Could you check a few things on this model? Use its own coordinates, in mm. A direction names the side the tool comes from. Give positions to 0.01 mm unless a question says otherwise; leave off trailing zeros. Write each loop counter-clockwise with the first axis right and the second up, starting at its lowest first coordinate (ties: lowest second). Pieces come first, ordered by that corner, then holes. Notation, with made-up numbers: (39.5, -32.5) -> (89.5, -32.5) arc R19 cw to (89.5, -5.5) -> close; hole circle Ø8 at (44.25, 2.5). An arc over 180 degrees is marked (long way). One line per question, with ' | ' between items.
from build123d import *
from build123d import SkipClean  # not in build123d's __all__

# Parameters (mm, degrees)
F0_R     = 2
F1_DEPTH = 2
F3_DEPTH = 1
F5_DEPTH = 5
F8_DEPTH = 8
F9_DEPTH = 8


with BuildPart() as f1:
    # F0 (on Top) → F1 (new body)
    with BuildSketch(Plane.XY):
        with BuildLine():
            ThreePointArc((-5, 0), (-3.5355339059, 3.5355339059), (0, 5))
            Line((0, 5), (0, 7))
            ThreePointArc((0, 7), (-4.9497474683, 4.9497474683), (-7, 0))
            Line((-7, 0), (-5, 0))
        make_face()
        with BuildLine():
            ThreePointArc((0, 5), (3.5355339059, 3.5355339059), (5, 0))
            Line((5, 0), (7, 0))
            ThreePointArc((7, 0), (4.9497474683, 4.9497474683), (0, 7))
            Line((0, 7), (0, 5))
        make_face()
        with BuildLine():
            Line((7, 0), (5, 0))
            ThreePointArc((5, 0), (3.5355339059, -3.5355339059), (0, -5))
            Line((0, -5), (0, -7))
            ThreePointArc((0, -7), (4.9497474683, -4.9497474683), (7, 0))
        make_face()
        with BuildLine():
            Line((0, -7), (0, -5))
            ThreePointArc((0, -5), (-3.5355339059, -3.5355339059), (-5, 0))
            Line((-5, 0), (-7, 0))
            ThreePointArc((-7, 0), (-4.9497474683, -4.9497474683), (0, -7))
        make_face()
        with BuildLine():
            ThreePointArc((0, -5), (3.5355339059, -3.5355339059), (5, 0))
            ThreePointArc((5, 0), (3.5355339059, 3.5355339059), (0, 5))
            ThreePointArc((0, 5), (-3.5355339059, 3.5355339059), (-5, 0))
            ThreePointArc((-5, 0), (-3.5355339059, -3.5355339059), (0, -5))
        make_face()
        Circle(F0_R, mode=Mode.SUBTRACT)
    extrude(amount=F1_DEPTH)

    # F2 (on face) → F3 (join)
    with BuildSketch(Plane.XY.offset(2)):
        with BuildLine():
            ThreePointArc((-5, 0), (-3.5355339059, 3.5355339059), (0, 5))
            Line((0, 5), (0, 7))
            ThreePointArc((0, 7), (-1.1928549598, 6.8976153158), (-2.3508156114, 6.5934562986))
            Line((-2.3508156114, 6.5934562986), (-6.5934562986, 2.3508156114))
            ThreePointArc((-6.5934562986, 2.3508156114), (-6.8976153158, 1.1928549598), (-7, 0))
            Line((-7, 0), (-5, 0))
        make_face()
        with BuildLine():
            Line((-6.5934562986, 2.3508156114), (-2.3508156114, 6.5934562986))
            ThreePointArc((-2.3508156114, 6.5934562986), (-4.9497474683, 4.9497474683), (-6.5934562986, 2.3508156114))
        make_face()
        with BuildLine():
            ThreePointArc((2.3508156114, -6.5934562986), (4.9497474683, -4.9497474683), (6.5934562986, -2.3508156114))
            Line((6.5934562986, -2.3508156114), (2.3508156114, -6.5934562986))
        make_face()
        with BuildLine():
            Line((7, 0), (5, 0))
            ThreePointArc((5, 0), (3.5355339059, -3.5355339059), (0, -5))
            Line((0, -5), (0, -7))
            ThreePointArc((0, -7), (1.1928549598, -6.8976153158), (2.3508156114, -6.5934562986))
            Line((2.3508156114, -6.5934562986), (6.5934562986, -2.3508156114))
            ThreePointArc((6.5934562986, -2.3508156114), (6.8976153158, -1.1928549598), (7, 0))
        make_face()
    with SkipClean():  # cleaning this boolean's faces spoils the solid; the shape is the same uncleaned
        extrude(amount=F3_DEPTH)

    # F4 (on face) → F5 (join)
    with BuildSketch(Plane.XY.offset(3)):
        with BuildLine():
            ThreePointArc((-5, 0), (-3.5355339059, 3.5355339059), (0, 5))
            Line((0, 5), (0, 7))
            ThreePointArc((0, 7), (-1.1928549598, 6.8976153158), (-2.3508156114, 6.5934562986))
            Line((-2.3508156114, 6.5934562986), (-6.5934562986, 2.3508156114))
            ThreePointArc((-6.5934562986, 2.3508156114), (-6.8976153158, 1.1928549598), (-7, 0))
            Line((-7, 0), (-5, 0))
        make_face()
        with BuildLine():
            Line((7, 0), (5, 0))
            ThreePointArc((5, 0), (3.5355339059, -3.5355339059), (0, -5))
            Line((0, -5), (0, -7))
            ThreePointArc((0, -7), (1.1928549598, -6.8976153158), (2.3508156114, -6.5934562986))
            Line((2.3508156114, -6.5934562986), (6.5934562986, -2.3508156114))
            ThreePointArc((6.5934562986, -2.3508156114), (6.8976153158, -1.1928549598), (7, 0))
        make_face()
    extrude(amount=F5_DEPTH)

    # F7 (on face) → F8 (join)
    with BuildSketch(Plane(origin=(4.472135955, -4.472135955, 0), x_dir=(0.7071067812, 0.7071067812, 0), z_dir=(0.7071067812, -0.7071067812, 0))):
        with BuildLine():
            Line((1.1523319194, 6.4602765995), (0, 5.5))
            Line((0, 5.5), (1.1523319194, 4.5397234005))
            ThreePointArc((1.1523319194, 4.5397234005), (1.4104073665, 4.9893621044), (1.5, 5.5))
            ThreePointArc((1.5, 5.5), (1.4104073665, 6.0106378956), (1.1523319194, 6.4602765995))
        make_face()
        with BuildLine():
            Line((0, 5.5), (-1.1523319194, 6.4602765995))
            ThreePointArc((-1.1523319194, 6.4602765995), (-1.5, 5.5), (-1.1523319194, 4.5397234005))
            Line((-1.1523319194, 4.5397234005), (0, 5.5))
        make_face()
        with BuildLine():
            ThreePointArc((1.1523319194, 6.4602765995), (0, 7), (-1.1523319194, 6.4602765995))
            Line((-1.1523319194, 6.4602765995), (0, 5.5))
            Line((0, 5.5), (1.1523319194, 6.4602765995))
        make_face()
        with BuildLine():
            Line((1.1523319194, 4.5397234005), (0, 5.5))
            Line((0, 5.5), (-1.1523319194, 4.5397234005))
            ThreePointArc((-1.1523319194, 4.5397234005), (0, 4), (1.1523319194, 4.5397234005))
        make_face()
    extrude(amount=F8_DEPTH)

    # F6 (on face) → F9 (join)
    with BuildSketch(Plane(origin=(-4.472135955, 4.472135955, 0), x_dir=(-0.7071067812, -0.7071067812, 0), z_dir=(-0.7071067812, 0.7071067812, 0))):
        with BuildLine():
            ThreePointArc((1.1523319194, 6.4602765995), (0, 7), (-1.1523319194, 6.4602765995))
            Line((-1.1523319194, 6.4602765995), (0, 5.5))
            Line((0, 5.5), (1.1523319194, 6.4602765995))
        make_face()
        with BuildLine():
            Line((1.1523319194, 6.4602765995), (0, 5.5))
            Line((0, 5.5), (1.1523319194, 4.5397234005))
            ThreePointArc((1.1523319194, 4.5397234005), (1.4104073665, 4.9893621044), (1.5, 5.5))
            ThreePointArc((1.5, 5.5), (1.4104073665, 6.0106378956), (1.1523319194, 6.4602765995))
        make_face()
        with BuildLine():
            Line((1.1523319194, 4.5397234005), (0, 5.5))
            Line((0, 5.5), (-1.1523319194, 4.5397234005))
            ThreePointArc((-1.1523319194, 4.5397234005), (0, 4), (1.1523319194, 4.5397234005))
        make_face()
        with BuildLine():
            Line((0, 5.5), (-1.1523319194, 6.4602765995))
            ThreePointArc((-1.1523319194, 6.4602765995), (-1.5, 5.5), (-1.1523319194, 4.5397234005))
            Line((-1.1523319194, 4.5397234005), (0, 5.5))
        make_face()
    extrude(amount=F9_DEPTH)


solid = f1.part
Q1. Imagine slicing it at B-B on x = 0.5. Please give me the cut outline in (y, z), and give its area (3 significant figures).
Answer below:
outline: (-6.98, 0) -> (-1.94, 0) -> (-1.94, 2) -> (-4.97, 2) -> (-4.97, 8) -> (-6.98, 8) -> close; (1.94, 0) -> (6.98, 0) -> (6.98, 2) -> (1.94, 2) -> close | area: 32.2 mm^2
Q2. Will these pins go through, and if not, where does the flat tip stop? pin 1 (1.6 mm diameter, centred on y = 6, z = 5.5, fed in from +X); pin 2 (2 mm diameter, centred on y = 3.5, z = 2.5, fed in from -X); pin 3 (0.6 mm diameter, centred on x = -6, z = 5.5, fed in from -Y).
Answer below:
pin 1: stops at x = 0 | pin 2: stops at x = -6.54 | pin 3: stops at y = 0
Q3. If I drill on line 1 along Z through (x, y) = (2.25, -3.5); line 2 along X through (y, z) = (0.25, 7.5); line 3 along Y through (x, z) = (1.25, 4.5), over which ranges is the centre line in solid material (lowest first)?
Answer below:
line 1: z = 0 to 2 | line 2: x = -7 to -4.99 | line 3: y = -6.89 to -4.84
Q4. On a 3-axis mill with a long thin cutter (end or side, diameter ignored), from which of +Z, -Z, +X, -X, +Y, -Y can I reach the whole of each face in a straight line? I mean faces 4 (the flat face through (0, 6, 5)), 5 (the flat face through (1, 2, 2)), 6 (the flat face through (-6, 0, 5)), 7 (the cylindrical face through (-4, 3, 5)). Say none if no direction works.
Answer below:
face 4: +Z, +X, +Y | face 5: +Z | face 6: +Z, -X, -Y | face 7: +Z, +X, -Y
Q5. Imagine slicing it at C-C on y = -1.5. Please give me the cut outline in (x, z), and give its area (3 significant figures).
Answer below:
outline: (-6.84, 0) -> (-1.32, 0) -> (-1.32, 2) -> (-6.84, 2) -> close; (1.32, 0) -> (6.84, 0) -> (6.84, 8) -> (4.77, 8) -> (4.77, 2) -> (1.32, 2) -> close | area: 34.5 mm^2
Q6. If we mould it in two halves opening along X, with no side actions, what happens to faces 1 (the flat face through (4.442, -4.502, 3.798)), 2 (the cylindrical face through (4, -3, 5)), 3 (the flat face through (-4.6, 4.6, 3))? For each: +X half, -X half, draft (parallel to the pull), parting line (faces both ways), or undercut.
Answer below:
face 1: undercut | face 2: -X half | face 3: draft
Q7. Imagine slicing it at A-A on z = 3.5. Please give me the cut outline in (x, y), and give its area (3 significant figures).
Answer below:
outline: (-7, 0) -> (-5, 0) arc R5 cw to (0, 5) -> (0, 7) arc R7 ccw to (-2.35, 6.59) -> (-6.59, 2.35) arc R7 ccw to start; (0, -7) arc R7 ccw to (2.35, -6.59) -> (6.59, -2.35) arc R7 ccw to (7, 0) -> (5, 0) arc R5 cw to (0, -5) -> close | area: 32.2 mm^2
Q8. Imagine slicing it at D-D on z = 1. Please give me the cut outline in (x, y), and give its area (3 significant figures).
Answer below:
outline: circle Ø14 at (0, 0); hole circle Ø4 at (0, 0) | area: 141 mm^2
